Design review of the part built by this model. Coordinates are the model's own, in mm. A direction names the side the tool comes from. Give positions to 0.01 mm unless a question says otherwise; leave off trailing zeros. Write each loop counter-clockwise with the first axis right and the second up, starting at its lowest first coordinate (ties: lowest second). Pieces come first, ordered by that corner, then holes. Notation, with made-up numbers: (39, 7.25) - (53, 7.25) arc R9 cw to (53, 21.25) - close; hole circle Ø11 at (12, 16.25). An arc over 180 degrees is marked (long way). Write each question's results on one line, items separated by ' | '. Start each with the question number.
from build123d import *

# Parameters (mm, degrees)
SKETCH_1_R          = 17
EXTRUDE_1_DEPTH     = 2
EXTRUDE_2_DEPTH     = 1
FILLET_1_R          = 1.55
FILLET_2_R          = 0.8
SKETCH_3_R          = 7
CUT_EXTRUDE_1_DEPTH = 25.22808302


with BuildPart() as part:
    # ｽｹｯﾁ1 → ﾎﾞｽ - 押し出し1 (new body)
    with BuildSketch(Plane.XY):
        Circle(SKETCH_1_R)
    extrude(amount=EXTRUDE_1_DEPTH)

    # ｽｹｯﾁ2 → ﾎﾞｽ - 押し出し2 (add)
    with BuildSketch(Plane.XY.offset(2)):
        with BuildLine():
            Line((-1.5, 14.422205102), (-1.5, 12.5))
            Line((-1.5, 12.5), (1.5, 12.5))
            Line((1.5, 12.5), (1.5, 14.422205102))
            ThreePointArc((1.5, 14.422205102), (0, 14.5), (-1.5, 14.422205102))
        make_face()
        with BuildLine():
            Line((1.5, 12.5), (-1.5, 12.5))
            Line((-1.5, 12.5), (-1.5, 14.422205102))
            ThreePointArc((-1.5, 14.422205102), (-9.708243919, -10.770329614), (14.5, 0))
            ThreePointArc((14.5, 0), (10.770329614, 9.708243919), (1.5, 14.422205102))
            Line((1.5, 14.422205102), (1.5, 12.5))
        make_face()
        with BuildLine():
            Line((-1.5, 16.5), (-1.5, 14.422205102))
            ThreePointArc((-1.5, 14.422205102), (0, 14.5), (1.5, 14.422205102))
            Line((1.5, 14.422205102), (1.5, 16.5))
            Line((1.5, 16.5), (-1.5, 16.5))
        make_face()
    extrude(amount=EXTRUDE_2_DEPTH)

    # ﾌｨﾚｯﾄ1
    fillet_1_edges = [part.edges().sort_by_distance(p)[0] for p in [
        (-1.5, 14.422205102, 2.5),
        (1.5, 14.422205102, 2.5),
    ]]
    fillet(fillet_1_edges, radius=FILLET_1_R)

    # ﾌｨﾚｯﾄ2
    fillet_2_edges = [part.edges().sort_by_distance(p)[0] for p in [
        (1.5, 16.5, 2.5),
        (-1.5, 16.5, 2.5),
    ]]
    fillet(fillet_2_edges, radius=FILLET_2_R)

    # ｽｹｯﾁ3 → ｶｯﾄ - 押し出し1 (cut, through all)
    with BuildSketch(Plane.XY.offset(3)):
        Circle(SKETCH_3_R)
    extrude(amount=-CUT_EXTRUDE_1_DEPTH, mode=Mode.SUBTRACT)


solid = part.part
Q1. Add section A-A on x = 0. State the section outline as (y, z) points, plus the area to 3 significant figures.
Q2. Add section D-D on y = -12. State the section outline as (x, z) points, plus the area to 3 significant figures.
Q3. For line 1 along Y through (x, z) = (0, 0.8); line 2 along Y through (x, z) = (2, 2.45); line 3 along X through (y, z) = (0.5, 2.7), list the stretches that pass through material, from the lowest coordinate up. Write a range as [from, to].
Q4. Machinability: for faces 1 (the face through (0, 16.5, 2.5)), 2 (the face through (-1.876, 14.745, 2.507)), 3 (the face through (1.876, 14.745, 2.507)), which of the approach directions +Z, -Z, +X, -X, +Y, -Y give a long, thin tool a straight path to every point of the face, cutting with its end or side? Answer none if there is none.
Q5. Insertion check: P1, Ø0.5, axis at x = 0, z = 2.5, coming from the +Y side. The pin has a flat end and moves straight along its axis. Give the tip position at first contact, or say it passes through.
Q6. Add section B-B on y = 6. State the section outline as (x, z) points.
Q7. Add section C-C on z = 0.8. State the section outline as (x, y) points, plus the area to 3 significant figures.
Q8. The part is to be moulded in two halves that separate along Y. For faces 4 (the face through (6.466, -2.681, 1.521)), 5 (the face through (9.139, 14.334, 0.986)), 6 (the face through (7, -13, 2)), say which applies: +Y half, -Y half, draft (parallel to the pull), parting line (faces both ways), or undercut.
Result:
1) outline: (-17, 0) - (-7, 0) - (-7, 3) - (-14.5, 3) - (-14.5, 2) - (-17, 2) - close; (7, 0) - (17, 0) - (17, 2) - (16.5, 2) - (16.5, 3) - (7, 3) - close | area: 57.0 mm²
2) outline: (-12.04, 0) - (12.04, 0) - (12.04, 2) - (8.14, 2) - (8.14, 3) - (-8.14, 3) - (-8.14, 2) - (-12.04, 2) - close | area: 64.4 mm²
3) line 1: y = [-17, -7], [7, 17] | line 2: y = [-14.36, -6.71], [6.71, 14.62] | line 3: x = [-14.49, -6.98], [6.98, 14.49]
4) face 1: +Z, +X, -X, +Y | face 2: +Z, -X, +Y | face 3: +Z, +X, +Y
5) P1: stops at y = 16.5
6) outline: (-15.91, 0) - (-3.61, 0) - (-3.61, 3) - (-13.2, 3) - (-13.2, 2) - (-15.91, 2) - close; (3.61, 0) - (15.91, 0) - (15.91, 2) - (13.2, 2) - (13.2, 3) - (3.61, 3) - close
7) outline: circle Ø34 at (0, 0); hole circle Ø14 at (0, 0) | area: 754 mm²
8) face 4: undercut | face 5: parting line | face 6: draft
